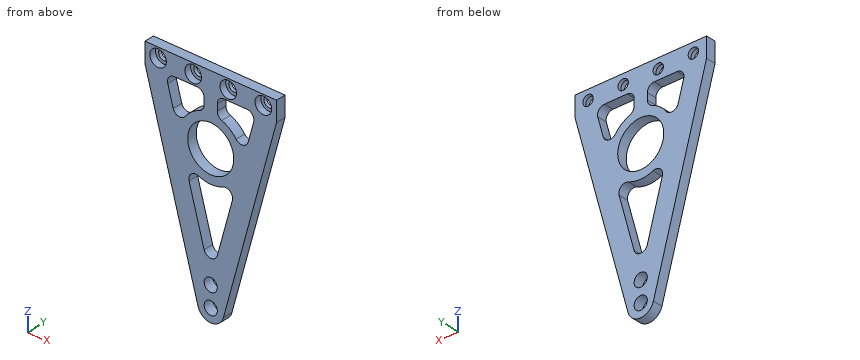
```python
from build123d import *

# Parameters (mm, degrees)
F0_R           = 11.1125
F1_DEPTH       = 4.7625
F3_DEPTH       = 4.7635
F4_R           = 3.302
F5_R           = 3.175
F6_DEPTH       = 4.7635
F8_D           = 4.9784
F8_CBORE_D     = 7.9756
F8_CBORE_DEPTH = 3.175


with BuildPart() as f1:
    # F0 (on Front) → F1 (new body)
    with BuildSketch(Plane.XZ):
        with BuildLine():
            Line((31.75, 29.791584), (31.75, 39.316584))
            Line((31.75, 39.316584), (-31.75, 39.316584))
            Line((-31.75, 39.316584), (-31.75, 29.791584))
            Line((-31.75, 29.791584), (-6.123568, -63.583015))
            ThreePointArc((-6.123568, -63.583015), (0, -68.252416), (6.123568, -63.583015))
            Line((6.123568, -63.583015), (31.75, 29.791584))
        make_face()
        with Locations((0, 6.017184)):
            Circle(F0_R, mode=Mode.SUBTRACT)
    extrude(amount=F1_DEPTH)

    # F2 (on face) → F3 (cut, through all)
    with BuildSketch(Plane.XZ.offset(4.7625)):
        with BuildLine():
            Line((-3.175, 29.791584), (-21.872793, 29.791584))
            Line((-21.872793, 29.791584), (-15.161242, 5.336816))
            ThreePointArc((-15.161242, 5.336816), (-12.011665, 15.293285), (-3.175, 20.857855))
            Line((-3.175, 20.857855), (-3.175, 29.791584))
        make_face()
        with BuildLine():
            Line((15.161242, 5.336816), (21.872793, 29.791584))
            Line((21.872793, 29.791584), (3.175, 29.791584))
            Line((3.175, 29.791584), (3.175, 20.857855))
            ThreePointArc((3.175, 20.857855), (12.011665, 15.293285), (15.161242, 5.336816))
        make_face()
        with BuildLine():
            Line((0, -49.905946), (13.384579, -1.13678))
            ThreePointArc((13.384579, -1.13678), (0, -9.159316), (-13.384579, -1.13678))
            Line((-13.384579, -1.13678), (0, -49.905946))
        make_face()
    extrude(amount=-F3_DEPTH, mode=Mode.SUBTRACT)

    # F4
    f4_edges = [f1.edges().sort_by_distance(p)[0] for p in [
        (-21.872793, -2.38125, 29.791584),
        (3.175, -2.38125, 29.791584),
        (-3.175, -2.38125, 29.791584),
        (21.872793, -2.38125, 29.791584),
        (3.175, -2.38125, 20.857855),
        (-3.175, -2.38125, 20.857855),
        (15.161242, -2.38125, 5.336816),
        (-15.161242, -2.38125, 5.336816),
        (-13.384579, -2.38125, -1.13678),
        (13.384579, -2.38125, -1.13678),
        (0, -2.38125, -49.905946),
    ]]
    fillet(f4_edges, radius=F4_R)

    # F5 (on face) → F6 (cut, through all)
    with BuildSketch(Plane.XZ.offset(4.7625)):
        with Locations((0, -61.902416)):
            Circle(F5_R)
        with Locations((0, -52.047216)):
            Circle(F5_R)
    extrude(amount=-F6_DEPTH, mode=Mode.SUBTRACT)

    # F8 (through all)
    with Locations(Plane.XZ.offset(4.7625)):
        with Locations((-25.4, 34.554084), (-8.4582, 34.554084), (8.4582, 34.554084), (25.4, 34.554084)):
            CounterBoreHole(F8_D / 2, F8_CBORE_D / 2, F8_CBORE_DEPTH)


solid = f1.part
```
Design review of the part built by this model. Coordinates are the model's own, in mm. Give positions to 0.01 mm unless a question says otherwise; leave off trailing zeros. Write each loop counter-clockwise with the first axis right and the second up, starting at its lowest first coordinate (ties: lowest second). Pieces come first, ordered by that corner, then holes.
(1) Add section D-D (y = -3). Give the number of separate pieces and of enclosed holes in the cut face, and give its area (3 significant figures).
Checked values:
separate pieces: 1
enclosed holes: 10
area: 2,670 mm2
(2) Add section A-A (x = 0). Give the boundary of the cut face in (y, z), and give its area (3 significant figures).
Checked values:
outline: (-4.76, -68.25) - (0, -68.25) - (0, -65.08) - (-4.76, -65.08) - close; (-4.76, -58.73) - (0, -58.73) - (0, -55.22) - (-4.76, -55.22) - close; (-4.76, -48.87) - (0, -48.87) - (0, -40.73) - (-4.76, -40.73) - close; (-4.76, -9.16) - (0, -9.16) - (0, -5.1) - (-4.76, -5.1) - close; (-4.76, 17.13) - (0, 17.13) - (0, 39.32) - (-4.76, 39.32) - close
area: 196 mm2
(3) Clearance check with flat-ended pins moving along their axes: pin 1 Ø2.5 at (y, z) = (-2.5, 25) entering from +X; pin 2 Ø1.6 at (y, z) = (-2.5, 25) entering from -X. State where each tip first meets the part, or that it passes through.
Checked values:
pin 1: stops at x = 30.78
pin 2: stops at x = -30.65
(4) Add section C-C (x = -25.4). Give the boundary of the cut face in (y, z), and give its area (3 significant figures).
Checked values:
outline: (-4.76, 6.65) - (0, 6.65) - (0, 32.06) - (-1.59, 32.06) - (-1.59, 30.57) - (-4.76, 30.57) - close; (-4.76, 38.54) - (-1.59, 38.54) - (-1.59, 37.04) - (0, 37.04) - (0, 39.32) - (-4.76, 39.32) - close
area: 122 mm2
(5) Wall thickness on line 1 along X through (y, z) = (-4.5, -29.5); line 2 along X through (y, z) = (-2.45, -16); line 3 along Y through (x, z) = (-29, 34): over which ranges is each line inside the solid? List them lowest first.
Checked values:
line 1: x = -15.48 to -5.6, 5.6 to 15.48
line 2: x = -19.18 to -9.31, 9.31 to 19.18
line 3: y = -1.59 to 0
(6) Add section B-B (z = 2). Give the boundary of the cut face in (x, y), and give its area (3 significant figures).
Checked values:
outline: (-24.12, -4.76) - (-10.36, -4.76) - (-10.36, 0) - (-24.12, 0) - close; (10.36, -4.76) - (24.12, -4.76) - (24.12, 0) - (10.36, 0) - close
area: 131 mm2
